Part model, mm, in its own coordinate system. Face numbers are marked on the shaded views. A direction names the side the tool comes from. Coordinates: 2 decimals unless noted, no trailing zeros. Loops run counter-clockwise (first coordinate to the right, second up) from the corner with the lowest first, then second, coordinate; pieces in that order, holes last. Notation, with made-up numbers: M 34.25,22.5 L 61.25,22.5 A26 cw 61.25,44.5 Z; hole C -16,39.5 d2. An arc over 180 degrees is marked long. Answer as a JSON object with one key per item and string values. Group by question number.
1. Saw through at A-A on z = 5. Write the cut outline in (x, y), then the cut area to 3 significant figures.
2. 3-axis set-ups, long thin cutter, end or side, ignore diameter. For the marked faces 5, 6 and 7: which of +Z, -Z, +X, -X, +Y, -Y reach the whole face in a straight line?
3. Saw through at B-B on y = 0. Write the cut outline in (x, z), then the cut area to 3 significant figures.
4. Mould opens along Z. For the marked faces 1, 2, 3 and 4 say: released by +Z, released by -Z, zero draft, split by the parting line, or undercut.
5. Saw through at C-C on x = 0. Write the cut outline in (y, z).
6. Drop flat-ended pins along their axis: pin 1 Ø6.5 at (x, y) = (3.5, 3) entering from +Z; pin 2 Ø5 at (x, y) = (-15.5, -15.5) entering from +Z; pin 3 Ø1 at (x, z) = (4.5, 22.5) entering from -Y; pin 4 Ø2.5 at (x, y) = (-15.5, 15.5) entering from +Z. Give the stop position or say it passes through.
7. Drill centre lines: L1, parallel to Y at x = -15.5, z = -11.25; L2, parallel to X at y = 14.5, z = -13; L3, parallel to Y at x = 15, z = 11. Where is each one in solid material? Low to high.
8. Saw through at D-D on y = 12.5. Write the cut outline in (x, z).
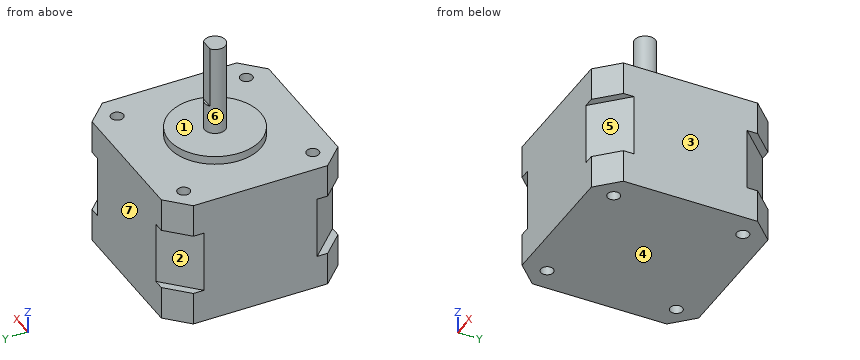
from build123d import *

# Parameters (mm, degrees)
F0_W      = 42.418
F0_H      = 42.418
F4_DEPTH  = 7.5
F5_SIZE   = 7.62
F7_DEPTH  = 8
F8_SIZE   = 5.08
F10_DEPTH = 8
F11_R     = 10.9982
F12_DEPTH = 2
F13_R     = 2.5
F14_DEPTH = 22
F16_DEPTH = 15
F17_R     = 1.5
F18_DEPTH = 6.35
F21_R     = 1.5
F22_DEPTH = 6.35


with BuildPart() as f4:
    # F0 (on Top) → F4 (new body, symmetric)
    with BuildSketch(Plane.XY):
        Rectangle(F0_W, F0_H)
    extrude(amount=F4_DEPTH, both=True)

    # F5
    f5_edges = [f4.edges().sort_by_distance(p)[0] for p in [
        (21.209, 21.209, 0),
        (-21.209, 21.209, 0),
        (-21.209, -21.209, 0),
        (21.209, -21.209, 0),
    ]]
    chamfer(f5_edges, length=F5_SIZE)

    # F6 (on face) → F7 (join)
    with BuildSketch(Plane.XY.offset(7.5)):
        Polygon((13.589, 21.209), (-13.589, 21.209), (-21.209, 13.589), (-21.209, -13.589), (-13.589, -21.209), (13.589, -21.209), (21.209, -13.589), (21.209, 13.589), align=None)
        Polygon((21.209, 21.209), (13.589, 21.209), (21.209, 13.589), align=None)
        Polygon((-13.589, 21.209), (-21.209, 21.209), (-21.209, 13.589), align=None)
        Polygon((-13.589, -21.209), (-21.209, -13.589), (-21.209, -21.209), align=None)
        Polygon((21.209, -21.209), (21.209, -13.589), (13.589, -21.209), align=None)
    extrude(amount=F7_DEPTH)

    # F8
    f8_edges = [f4.edges().sort_by_distance(p)[0] for p in [
        (21.209, 21.209, 11.5),
        (-21.209, 21.209, 11.5),
        (-21.209, -21.209, 11.5),
        (21.209, -21.209, 11.5),
    ]]
    chamfer(f8_edges, length=F8_SIZE)

    # F9 (on face) → F10 (join)
    with BuildSketch(Plane(origin=(0, 0, -7.5), x_dir=(1, 0, 0), z_dir=(0, 0, -1))):
        Polygon((-13.589, 21.209), (-16.129, 21.209), (-21.209, 16.129), (-21.209, 13.589), align=None)
        Polygon((16.129, 21.209), (13.589, 21.209), (21.209, 13.589), (21.209, 16.129), align=None)
        Polygon((21.209, -16.129), (21.209, -13.589), (13.589, -21.209), (16.129, -21.209), align=None)
        Polygon((-13.589, -21.209), (-21.209, -13.589), (-21.209, -16.129), (-16.129, -21.209), align=None)
        Polygon((13.589, 21.209), (-13.589, 21.209), (-21.209, 13.589), (-21.209, -13.589), (-13.589, -21.209), (13.589, -21.209), (21.209, -13.589), (21.209, 13.589), align=None)
    extrude(amount=F10_DEPTH)

    # F11 (on face) → F12 (join)
    with BuildSketch(Plane.XY.offset(15.5)):
        Circle(F11_R)
    extrude(amount=F12_DEPTH)

    # F13 (on face) → F14 (join)
    with BuildSketch(Plane.XY.offset(17.5)):
        Circle(F13_R)
    extrude(amount=F14_DEPTH)

    # F15 (on face) → F16 (cut)
    with BuildSketch(Plane.XY.offset(39.5)):
        with BuildLine():
            Line((2.6203631624, 2.9334036984), (-2.6333660554, 2.9334036984))
            Line((-2.6333660554, 2.9334036984), (-2.6333660554, 2))
            Line((-2.6333660554, 2), (-1.5, 2))
            ThreePointArc((-1.5, 2), (0, 2.5), (1.5, 2))
            Line((1.5, 2), (2.6203631624, 2))
            Line((2.6203631624, 2), (2.6203631624, 2.9334036984))
        make_face()
        with BuildLine():
            ThreePointArc((1.5, 2), (0, 2.5), (-1.5, 2))
            Line((-1.5, 2), (1.5, 2))
        make_face()
    extrude(amount=-F16_DEPTH, mode=Mode.SUBTRACT)

    # F17 (on face) → F18 (cut)
    with BuildSketch(Plane.XY.offset(15.5)):
        with Locations((-15.5, 15.5)):
            Circle(F17_R)
        with Locations((15.5, 15.5)):
            Circle(F17_R)
        with Locations((15.5, -15.5)):
            Circle(F17_R)
        with Locations((-15.5, -15.5)):
            Circle(F17_R)
    extrude(amount=-F18_DEPTH, mode=Mode.SUBTRACT)


with BuildPart() as f19_1:
    # F19: copy of F4
    add(f4.part)


with BuildPart() as f4_1:
    add(f4.part)

    # F21 (on face) → F22 (cut)
    with BuildSketch(Plane(origin=(0, 0, -15.5), x_dir=(1, 0, 0), z_dir=(0, 0, -1))):
        with Locations((-15.5, 15.5)):
            Circle(F21_R)
        with Locations((15.5, 15.5)):
            Circle(F21_R)
        with Locations((15.5, -15.5)):
            Circle(F21_R)
        with Locations((-15.5, -15.5)):
            Circle(F21_R)
    extrude(amount=-F22_DEPTH, mode=Mode.SUBTRACT)


solid = f4_1.part
Outcome:
{
 "1": {"outline": "M -21.21,-13.59 L -13.59,-21.21 L 13.59,-21.21 L 21.21,-13.59 L 21.21,13.59 L 13.59,21.21 L -13.59,21.21 L -21.21,13.59 Z", "area": "1,680 mm²"},
 "2": {"face 5": "+X, -Y", "face 6": "+Z", "face 7": "+Z, -Z, +X, -X, +Y"},
 "3": {"outline": "M -21.21,-15.5 L 21.21,-15.5 L 21.21,15.5 L 11,15.5 L 11,17.5 L 2.5,17.5 L 2.5,39.5 L -2.5,39.5 L -2.5,17.5 L -11,17.5 L -11,15.5 L -21.21,15.5 Z", "area": "1,470 mm²"},
 "4": {"face 1": "released by +Z", "face 2": "undercut", "face 3": "zero draft", "face 4": "released by -Z"},
 "5": {"outline": "M -21.21,-15.5 L 21.21,-15.5 L 21.21,15.5 L 11,15.5 L 11,17.5 L 2.5,17.5 L 2.5,24.5 L 2,24.5 L 2,39.5 L -2.5,39.5 L -2.5,17.5 L -11,17.5 L -11,15.5 L -21.21,15.5 Z"},
 "6": {"pin 1": "stops at z = 39.5", "pin 2": "stops at z = 15.5", "pin 3": "passes through", "pin 4": "stops at z = 9.15"},
 "7": {"L1": "y = -21.21 to -17, -14 to 14, 17 to 21.21", "L2": "x = -21.21 to -16.62, -14.38 to 14.38, 16.62 to 21.21", "L3": "y = -21.21 to -16.91, -14.09 to 14.09, 16.91 to 21.21"},
 "8": {"outline": "M -21.21,-15.5 L 21.21,-15.5 L 21.21,15.5 L -21.21,15.5 Z"}
}
